Can you work these out from the drawing? Everything is in mm from the part's minimum corner. A direction names the side the tool comes from. Coordinates: 2 decimals unless noted, no trailing zeros. Loops run counter-clockwise (first coordinate to the right, second up) from the corner with the lowest first, then second, coordinate; pieces in that order, holes last. Notation, with made-up numbers: M -10,56.5 L 13,56.5 A14 cw 13,80.5 Z; hole C 63,-24 d3. An arc over 180 degrees is marked long. Use CSV: the item, a comma, the result in double quotes. Start each with the question number.
Q1. If we section it at A-A (y = 173): Please give me the cut outline in (x, z).
Q2. For pin 1 Ø11.5 at (y, z) = (9.76, 29.27) entering from +X; pin 2 Ø1.5 at (y, z) = (74.5, 23.5) entering from +X; pin 3 Ø14.5 at (x, y) = (34.35, 11.45) entering from +Z, each with a flat end and sliding along its axis, tell me the tip position at first contact or that it passes through.
Q3. If we section it at C-C (x = 24): Please give me the cut outline in (y, z).
Q4. Please list where these lines run through material, in increasing order: probe 1 along X at (y, z) = (111, 35); probe 2 along Y at (x, z) = (30, 12) (1 decimal). Write a range as [from, to].
Q5. If we section it at B-B (z = 27.5): Please give me the cut outline in (x, y) (1 decimal).
Q6. Which directions (+Z, -Z, +X, -X, +Y, -Y) give clear straight access to the entire face, cutting with the end or side of a thin tool? Please do the marked faces 1 and 2.
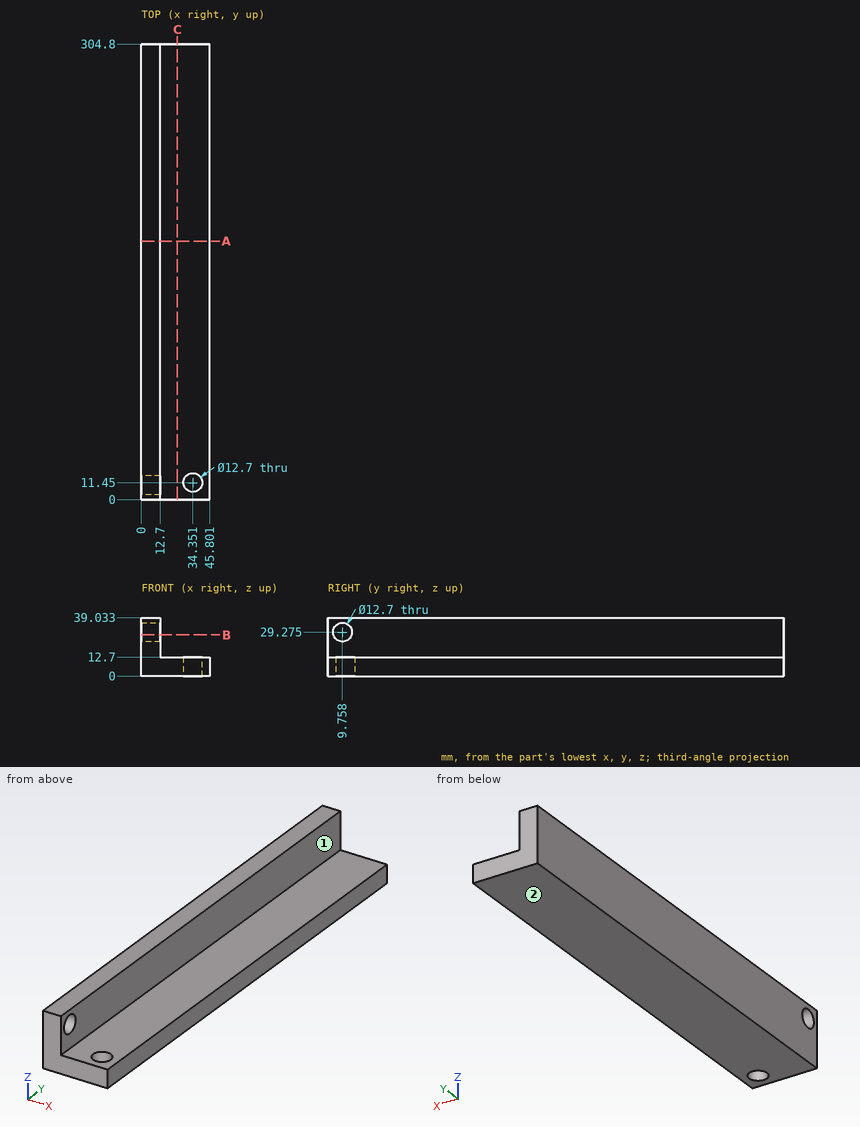
Results below:
1,outline,"M 0,0 L 45.8,0 L 45.8,12.7 L 12.7,12.7 L 12.7,39.03 L 0,39.03 Z"
2,pin 1,"through"
2,pin 2,"x = 12.7"
2,pin 3,"z = 12.7"
3,outline,"M 0,0 L 304.8,0 L 304.8,12.7 L 0,12.7 Z"
4,probe 1,"[0, 12.7]"
4,probe 2,"[0, 6.8], [16.1, 304.8]"
5,outline,"M 0,0 L 12.7,0 L 12.7,3.7 L 0,3.7 Z; M 0,15.9 L 12.7,15.9 L 12.7,304.8 L 0,304.8 Z"
6,face 1,"+Z, +X, +Y, -Y"
6,face 2,"-Z, +X, -X, +Y, -Y"
